```python
from build123d import *

# Parameters (mm, degrees)
SKETCH2_W           = 54
SKETCH2_H           = 30
BOSS_EXTRUDE1_DEPTH = 3
BOSS_EXTRUDE2_DEPTH = 10
BOSS_EXTRUDE4_DEPTH = 3
BOSS_EXTRUDE5_DEPTH = 10
BOSS_EXTRUDE3_DEPTH = 7


with BuildPart() as part:
    # Sketch2 → Boss-Extrude1 (new body)
    with BuildSketch(Plane(origin=(0, 0, 0), x_dir=(1, 0, 0), z_dir=(0, 1, 0))):
        Polygon((-55, 12), (-44, 12), (-44, -12), (-55, -12), (-55, -14), (-44, -22), (44, -22), (55, -14), (55, -12), (44, -12), (44, 12), (55, 12), (55, 14), (44, 22), (-44, 22), (-55, 14), align=None)
        with Locations((-14, 0)):
            Rectangle(SKETCH2_W, SKETCH2_H, mode=Mode.SUBTRACT)
    extrude(amount=BOSS_EXTRUDE1_DEPTH)

    # Sketch3 → Boss-Extrude2 (add)
    with BuildSketch(Plane(origin=(0, 3, 0), x_dir=(1, 0, 0), z_dir=(0, 1, 0))):
        Polygon((13, 20), (-44, 20), (-44, 12), (-55, 12), (-55, 14), (-44, 22), (13, 22), align=None)
        Polygon((-44, -12), (-44, -20), (13, -20), (13, -22), (-44, -22), (-55, -14), (-55, -12), align=None)
        Polygon((44, 12), (44, 22), (55, 14), (55, 12), align=None)
        Polygon((44, -22), (55, -14), (55, -12), (44, -12), align=None)
    extrude(amount=BOSS_EXTRUDE2_DEPTH)

    # Sketch5 → Boss-Extrude4 (add)
    with BuildSketch(Plane(origin=(0, 3, 0), x_dir=(1, 0, 0), z_dir=(0, 1, 0))):
        Polygon((13, -22), (44, -22), (33.5, -31), (23.5, -31), align=None)
        Polygon((44, 22), (13, 22), (23.5, 31), (33.5, 31), align=None)
    extrude(amount=-BOSS_EXTRUDE4_DEPTH)

    # Sketch6 → Boss-Extrude5 (add)
    with BuildSketch(Plane(origin=(0, 3, 0), x_dir=(1, 0, 0), z_dir=(0, 1, 0))):
        Polygon((21.166666667, -29), (23.5, -31), (33.5, -31), (35.833333333, -29), align=None)
        Polygon((35.833333333, 29), (33.5, 31), (23.5, 31), (21.166666667, 29), align=None)
    extrude(amount=BOSS_EXTRUDE5_DEPTH)

    # Sketch4 → Boss-Extrude3 (add)
    with BuildSketch(Plane.XZ):
        Polygon((13, 1.5), (13, -1.5), (27, -1.5), (27, -31), (30, -31), (30, -1.5), (44, -1.5), (44, 1.5), (30, 1.5), (30, 31), (27, 31), (27, 1.5), align=None)
    extrude(amount=BOSS_EXTRUDE3_DEPTH)


solid = part.part
```
Build history of the part. All positions in model axes, mm. A direction names the side the tool comes from. Coordinates: 2 decimals unless noted, no trailing zeros. Order: outer loops, then holes, each group sorted by start corner. A loop starts at its lowest first (then second) coordinate and runs counter-clockwise, first axis right, second up. Notation, with made-up numbers: (-16.5, 26) -> (-0.5, 26) arc R26 cw to (-0.5, 57) -> close; hole circle Ø1 at (77.5, 65). An arc over 180 degrees is marked (long way). Answer in a Markdown table with one row per item. Add a question column.
Q1. Band-saw the part on D-D, the plane y = 7.5. Give the number of separate pieces and of enclosed holes in the cut face, then the cut area to 3 significant figures.
Q2. Which spindle directions (+Z, -Z, +X, -X, +Y, -Y) get a long thin tool onto all of the face, cutting with end or side? Do faces 1 (the face through (20, -3, 1.5)), 2 (the face through (13, 8, 21)), 3 (the face through (-15, 8, -20)), 4 (the face through (-44, 1, 0)). Say none if no direction does.
Q3. Drop flat-ended pins along their axis: pin 1 (2.5 mm diameter, centred on y = 1, z = 5, fed in from +X); pin 2 (1.5 mm diameter, centred on x = -17.5, y = 1, fed in from -Z); pin 3 (6 mm diameter, centred on y = 5, z = -19.5, fed in from -X). Give the stop position or say it passes through.
Q4. Band-saw the part on A-A, the plane z = 6. List the corners of the cut face in (x, y), then the cut area to 3 significant figures.
Q5. Wall check: line 1 along X through (y, z) = (0.75, 14); line 2 along X through (y, z) = (0.5, 8.5); line 3 along Z through (x, y) = (-5.5, 1.5). Give the ranges that are in metal, low to high. Write a range as [from, to].
Q6. Band-saw the part on C-C, the plane y = -4. List the corners of the cut face in (x, z).
Q7. Mould opens along Z. For faces 5 (the face through (27, -3, -16)), 6 (the face through (29, 8, 29)), 7 (the face through (44, 0, 0)), 8 (the face through (-16, 6, 22)) say: +Z half, -Z half, draft (parallel to the pull), parting line (faces both ways), or undercut.
Q8. Band-saw the part on B-B, the plane x = -9.5. List the corners of the cut face in (y, z), then the cut area to 3 significant figures.
Answers follow:
| question | item | result |
|---|---|---|
| 1 | separate pieces | 6 |
| 1 | enclosed holes | 0 |
| 1 | area | 541 mm^2 |
| 2 | face 1 | +Z, -X, -Y |
| 2 | face 2 | +Z, -Z, +Y |
| 2 | face 3 | +Y |
| 2 | face 4 | -X, +Y, -Y |
| 3 | pin 1 | x = 44 |
| 3 | pin 2 | z = -22 |
| 3 | pin 3 | x = -51.56 |
| 4 | outline | (-44, 0) -> (-41, 0) -> (-41, 3) -> (-44, 3) -> close; (13, 0) -> (27, 0) -> (27, -7) -> (30, -7) -> (30, 0) -> (44, 0) -> (44, 3) -> (13, 3) -> close |
| 4 | area | 123 mm^2 |
| 5 | line 1 | [-55, -41], [13, 55] |
| 5 | line 2 | [-44, -41], [13, 44] |
| 5 | line 3 | [-22, -15], [15, 22] |
| 6 | outline | (13, -1.5) -> (27, -1.5) -> (27, -31) -> (30, -31) -> (30, -1.5) -> (44, -1.5) -> (44, 1.5) -> (30, 1.5) -> (30, 31) -> (27, 31) -> (27, 1.5) -> (13, 1.5) -> close |
| 7 | face 5 | draft |
| 7 | face 6 | undercut |
| 7 | face 7 | undercut |
| 7 | face 8 | +Z half |
| 8 | outline | (0, -22) -> (13, -22) -> (13, -20) -> (3, -20) -> (3, -15) -> (0, -15) -> close; (0, 15) -> (3, 15) -> (3, 20) -> (13, 20) -> (13, 22) -> (0, 22) -> close |
| 8 | area | 82.0 mm^2 |
